Autodesk Inventor part; units mm, degrees
ref_plane "Work Plane1" through (39, 0, 0) normal (1, 0, 0) x (0, 1, 0)
ref_plane "XZ Plane" through (0, 0, 0) normal (0, 1, 0) x (-1, 0, 0)
ref_plane "XY Plane" through (0, 0, 0) normal (0, 0, 1) x (1, 0, 0)
sketch "Sketch1" plane through (0, 0, 0) normal (0, 0, 1) x (1, 0, 0)
  line L0 (-522.2408, 82.6105) -> (-274.5908, 82.6105) construction
  line L1 (-274.5908, 82.6105) -> (-274.5908, -141.3329) construction
  line L2 (-274.5908, -141.3329) -> (-522.2408, -141.3329) construction
  line L3 (-522.2408, -141.3329) -> (-522.2408, 82.6105) construction
  circle A0 centre (0, 0) radius 25
  circle A1 centre (0, 0) radius 39
  dimension "d7" = 50
  dimension "d8" = 78
extrude "Extrusion1" add sketch "Sketch1" along normal blind 10
ref_plane "Work Plane1" through (39, 0, 0) normal (1, 0, 0) x (0, 1, 0)
sketch "Sketch2" plane through (39, 0, 0) normal (1, 0, 0) x (0, 1, 0)
  line L0 (39, 10) -> (-39, 10)
  line L1 (3.0144, 10) -> (-6.9856, 10)
  line L2 (-6.9856, 10) -> (-6.9856, 0)
  line L3 (-6.9856, 0) -> (3.0144, 0)
  line L4 (3.0144, 0) -> (3.0144, 10)
  point P0 (0, 0)
  dimension "d13" = 10
  dimension "d14" = 10
extrude "Extrusion2" add sketch "Sketch2" along normal blind 5 and the other way blind 5
pattern_circular "Circular Pattern1" count 16 over 360 about axis through (0, 0, 0) along (0, 0, 1) of "Extrusion2"
properties part number "cad@36"
Design review of the part built by this model. Coordinates are the model's own, in mm. A direction names the side the tool comes from. Round coordinates to 2 decimals unless told otherwise and drop trailing zeros. Order: outer loops, then holes, each group sorted by start corner. A loop starts at its lowest first (then second) coordinate and runs counter-clockwise, first axis right, second up.
1) Consider section A-A (x = 0). State the section outline as (y, z) points.
The answers:
outline: (-44, 0) - (-25, 0) - (-25, 10) - (-44, 10) - close; (25, 0) - (44, 0) - (44, 10) - (25, 10) - close
2) For L1, parallel to Y at x = 0, z = 6; L2, parallel to Y at x = 22.5, z = 5.75; L3, parallel to Y at x = -35.5, z = 6.5, list the stretches that pass through material, from the lowest coordinate up.
The answers:
L1: y = -44 to -25, 25 to 44
L2: y = -32.38 to -10.9, 10.9 to 31.86, 36.07 to 38.31
L3: y = -26.73 to -25.62, -17.97 to 22.27
3) Draft analysis for pull direction X (two halves, no side actions). For faces 5 (the flat face through (39.41, -13.06, 4.93)), 6 (the flat face through (-40.687, -9.292, 5.07)), 7 (the flat face through (-9.292, 40.687, 5.07)), state which applies: released by +X, released by -X, zero draft, split by the parting line, or undercut.
The answers:
face 5: released by +X
face 6: released by -X
face 7: undercut
4) Clearance check with flat-ended pins moving along their axes: pin 1 Ø1.5 at (x, z) = (-41, 4) entering from -Y; pin 2 Ø5 at (x, z) = (-21.5, 6) entering from +Y; pin 3 Ø1.7 at (y, z) = (42, 3.5) entering from +X. State where each tip first meets the part, or that it passes through.
The answers:
pin 1: stops at y = -17.81
pin 2: stops at y = 39.76
pin 3: stops at x = 15.63
5) Machinability: for faces 1 (the flat face through (-27.147, -31.41, 4.93)), 2 (the flat face through (-31.41, 27.147, 4.93)), 3 (the flat face through (40.687, 9.292, 5.07)), 4 (the cylindrical face through (23.274, 31.294, 4.93)), which of the approach directions +Z, -Z, +X, -X, +Y, -Y give a long, thin tool a straight path to every point of the face, cutting with its end or side? Answer none if there is none.
The answers:
face 1: +Z, -Z, -Y
face 2: +Z, -Z, -X
face 3: +Z, -Z, +X
face 4: +Z, -Z
